from build123d import *

# Parameters (mm, degrees)
SKETCH1_W            = 7.8
SKETCH1_H            = 9.6
BOSS_EXTRUDE1_DEPTH  = 15.8
SKETCH2_R            = 2.4
BOSS_EXTRUDE2_DEPTH  = 1.6
LPATTERN1_COUNT      = 2
LPATTERN1_PITCH      = 8
LPATTERN1_COUNT_DIR2 = 4
LPATTERN1_PITCH_DIR2 = 8
SHELL1_T             = -1.2
SKETCH5_R            = 1.5
BOSS_EXTRUDE4_DEPTH  = 8.2


with BuildPart() as part:
    # Sketch1 → Boss-Extrude1 (new body)
    with BuildSketch(Plane.XY):
        with Locations((3.9, 4.8)):
            Rectangle(SKETCH1_W, SKETCH1_H)
    extrude(amount=-BOSS_EXTRUDE1_DEPTH)

    # Sketch2 → Boss-Extrude2 (add)
    with BuildSketch(Plane(origin=(0, 9.6, 0), x_dir=(1, 0, 0), z_dir=(0, 1, 0))):
        with Locations(Location((3.9, 3.9, 0), (0, 0, 270))):
            Circle(SKETCH2_R)
    boss_extrude2 = extrude(amount=BOSS_EXTRUDE2_DEPTH)

    # LPattern1: Boss-Extrude2 2 × 4, 6 skipped
    with Locations(*[(-j * LPATTERN1_PITCH_DIR2, 0, -i * LPATTERN1_PITCH) for i in range(LPATTERN1_COUNT) for j in range(LPATTERN1_COUNT_DIR2) if (i, j) not in ((0, 0), (0, 1), (0, 2), (0, 3), (1, 1), (1, 2), (1, 3))]):
        add(boss_extrude2)

    # Shell1
    shell1_openings = [part.faces().sort_by_distance(p)[0] for p in [
        (3.9, 0, -7.9),
    ]]
    offset(amount=SHELL1_T, openings=shell1_openings, kind=Kind.INTERSECTION)

    # Sketch5 → Boss-Extrude4 (add)
    with BuildSketch(Plane.XZ.offset(-8.4)):
        with Locations(Location((3.9, -7.9, 0), (0, 0, 90))):
            Circle(SKETCH5_R)
    extrude(amount=BOSS_EXTRUDE4_DEPTH)


solid = part.part
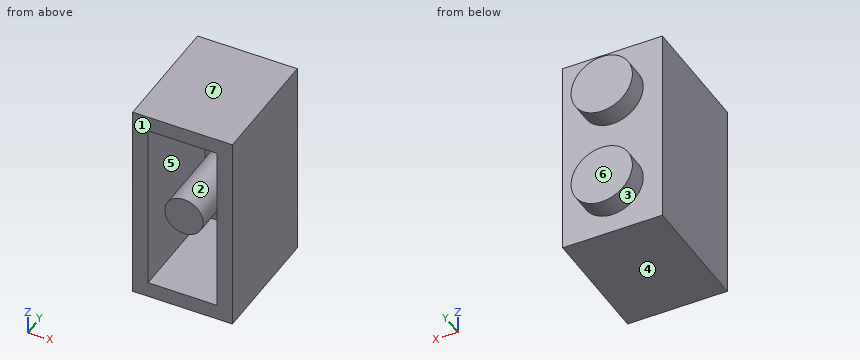
CAD build for the part. Positions are in the model's coordinates, mm. Face numbers are marked on the shaded views. A direction names the side the tool comes from. Coordinates: 2 decimals unless noted, no trailing zeros. Write each loop counter-clockwise with the first axis right and the second up, starting at its lowest first coordinate (ties: lowest second). Pieces come first, ordered by that corner, then holes. Notation, with made-up numbers: (87.5, 22) - (99.5, 22) arc R20 cw to (99.5, 34) - close; hole circle Ø7 at (55.5, 44.25). An arc over 180 degrees is marked (long way). Use a Markdown table: item, result. Add a question column.
Item 1: Band-saw the part on C-C, the plane y = 9.25. Give the cut face in (x, z), and give its area (3 significant figures).
Item 2: Band-saw the part on A-A, the plane y = 5. Give the cut face in (x, z).
Item 3: Band-saw the part on B-B, the plane z = -11.9. Give the cut face in (x, y).
Item 4: Flat gauge pins, fed straight in: pin 1 (1.2 mm diameter, centred on x = 4.5, z = -3.5, fed in from -Y); pin 2 (1.5 mm diameter, centred on x = 4, z = -8, fed in from -Y); pin 3 (0.7 mm diameter, centred on x = 4, z = -11.5, fed in from -Y). Where does each tip first touch, or does it go through?
Item 5: Band-saw the part on D-D, the plane x = 3.9. Give the cut face in (y, z).
Item 6: Drill centre lines: L1, parallel to Z at x = 3.9, y = 8.85; L2, parallel to Z at x = 4, y = 1.75; L3, parallel to X at y = 0.75, z = -13.25. Where is each one in solid material? Low to high. Write a range as from..to.
Item 7: 3-axis set-ups, long thin cutter, end or side, ignore diameter. For the marked faces 1, 2 and 3: which of +Z, -Z, +X, -X, +Y, -Y reach the whole face in a straight line?
Item 8: Mould opens along Z. For the marked faces 4, 5, 6 and 7 say: pulls with the +Z half, pulls with the -Z half, needs draft (parallel to the pull), parting line crosses it, or undercut.
Numbers:
| question | item | result |
|---|---|---|
| 1 | outline | (0, -15.8) - (7.8, -15.8) - (7.8, 0) - (0, 0) - close; hole circle Ø2.4 at (3.9, -11.9); hole circle Ø2.4 at (3.9, -3.9) |
| 1 | area | 114 mm2 |
| 2 | outline | (0, -15.8) - (7.8, -15.8) - (7.8, 0) - (0, 0) - close; circle Ø3 at (3.9, -7.9); hole (1.2, -14.6) - (6.6, -14.6) - (6.6, -1.2) - (1.2, -1.2) - close |
| 3 | outline | (0, 0) - (1.2, 0) - (1.2, 8.4) - (2.7, 8.4) - (2.7, 10) - (5.1, 10) - (5.1, 8.4) - (6.6, 8.4) - (6.6, 0) - (7.8, 0) - (7.8, 9.6) - (6.3, 9.6) - (6.3, 11.2) - (1.5, 11.2) - (1.5, 9.6) - (0, 9.6) - close |
| 4 | pin 1 | y = 8.4 |
| 4 | pin 2 | y = 0.2 |
| 4 | pin 3 | y = 10 |
| 5 | outline | (0, -15.8) - (9.6, -15.8) - (9.6, -14.3) - (11.2, -14.3) - (11.2, -9.5) - (9.6, -9.5) - (9.6, -6.3) - (11.2, -6.3) - (11.2, -1.5) - (9.6, -1.5) - (9.6, 0) - (0, 0) - (0, -1.2) - (8.4, -1.2) - (8.4, -2.7) - (10, -2.7) - (10, -5.1) - (8.4, -5.1) - (8.4, -6.4) - (0.2, -6.4) - (0.2, -9.4) - (8.4, -9.4) - (8.4, -10.7) - (10, -10.7) - (10, -13.1) - (8.4, -13.1) - (8.4, -14.6) - (0, -14.6) - close |
| 6 | L1 | -15.8..-13.1, -10.7..-5.1, -2.7..0 |
| 6 | L2 | -15.8..-14.6, -9.4..-6.4, -1.2..0 |
| 6 | L3 | 0..1.2, 6.6..7.8 |
| 7 | face 1 | +Z, -Z, +X, -X, -Y |
| 7 | face 2 | -Y |
| 7 | face 3 | +Y |
| 8 | face 4 | pulls with the -Z half |
| 8 | face 5 | undercut |
| 8 | face 6 | needs draft |
| 8 | face 7 | pulls with the +Z half |
